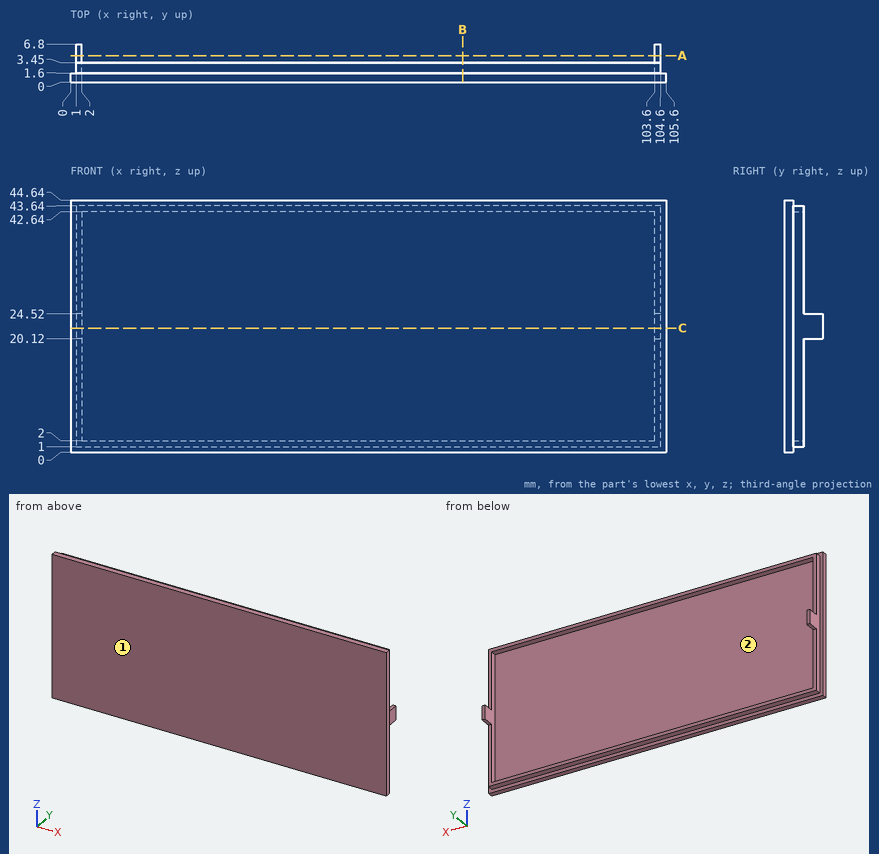
Could you check a few things on this drawing? It's one solid part, dimensions in mm from its lowest x, y, z. Give positions to 0.01 mm unless a question says otherwise; leave off trailing zeros. Loops run counter-clockwise (first coordinate to the right, second up) from the corner with the lowest first, then second, coordinate; pieces in that order, holes last. Notation, with made-up numbers: M 22.25,25.5 L 48.25,25.5 A14 cw 48.25,46.5 Z; hole C 7.25,-2.5 d2. An arc over 180 degrees is marked long. One line per question, with ' | ' between items. Start each with the question number.
Q1. If we section it at B-B (x = 69.5): Please give me the cut outline in (y, z).
Q2. If I drill on line 1 (Z direction, x = 66.5, y = 2); line 2 (X direction, y = 2.75, z = 27); line 3 (Y direction, x = 68, z = 31), over which ranges is the centre line in solid material (lowest first)? Write a range as from..to.
Q3. If we mould it in two halves opening along X, with no side actions, what happens to the marked faces 1 and 2? For each: +X half, -X half, draft (parallel to the pull), parting line (faces both ways), or undercut.
Q4. For pin 1 Ø2.5 at (y, z) = (3, 18) entering from -X; pin 2 Ø1.5 at (x, y) = (48, 2.5) entering from +Z; pin 3 Ø12 at (x, z) = (22.5, 10.5) entering from +Y; pin 4 Ø1.6 at (y, z) = (4.5, 14.5) entering from -X, each with a flat end and sliding along its axis, tell me the tip position at first contact or that it passes through.
Q5. If we section it at C-C (z = 22): Please give me the cut outline in (x, y).
Q6. If we section it at A-A (y = 4.75): Please give me the cut outline in (x, z), plus the area to 3 significant figures.
Computed:
1) outline: M 0,0 L 1.6,0 L 1.6,1 L 3.45,1 L 3.45,2 L 1.6,2 L 1.6,42.64 L 3.45,42.64 L 3.45,43.64 L 1.6,43.64 L 1.6,44.64 L 0,44.64 Z
2) line 1: z = 1..2, 42.64..43.64 | line 2: x = 1..2, 103.6..104.6 | line 3: y = 0..1.6
3) face 1: draft | face 2: undercut
4) pin 1: stops at x = 1 | pin 2: stops at z = 43.64 | pin 3: stops at y = 1.6 | pin 4: passes through
5) outline: M 0,0 L 105.6,0 L 105.6,1.6 L 104.6,1.6 L 104.6,6.8 L 103.6,6.8 L 103.6,1.6 L 2,1.6 L 2,6.8 L 1,6.8 L 1,1.6 L 0,1.6 Z
6) outline: M 1,20.12 L 2,20.12 L 2,24.52 L 1,24.52 Z; M 103.6,20.12 L 104.6,20.12 L 104.6,24.52 L 103.6,24.52 Z | area: 8.80 mm²
